from build123d import *

# Parameters (mm, degrees)
CROQUIS1_R              = 7.9
SALIENTE_EXTRUIR1_DEPTH = 7
CROQUIS2_R              = 6
SALIENTE_EXTRUIR2_DEPTH = 7.5
CROQUIS3_R              = 7.9
SALIENTE_EXTRUIR3_DEPTH = 1.5
CROQUIS4_R              = 4
CORTAR_EXTRUIR1_DEPTH   = 20.514609912
CROQUIS5_W              = 1.25
CROQUIS5_H              = 7.901
MATRIZC1_COUNT          = 2
MATRIZC1_ANGLE          = 90


with BuildPart() as part:
    # Croquis1 → Saliente-Extruir1 (new body)
    with BuildSketch(Plane(origin=(0, 0, 0), x_dir=(1, 0, 0), z_dir=(0, 1, 0))):
        with Locations(Location((0, 0, 0), (0, 0, 270))):
            Circle(CROQUIS1_R)
    extrude(amount=SALIENTE_EXTRUIR1_DEPTH)

    # Croquis2 → Saliente-Extruir2 (add)
    with BuildSketch(Plane(origin=(0, 7, 0), x_dir=(1, 0, 0), z_dir=(0, 1, 0))):
        with Locations(Location((0, 0, 0), (0, 0, 270))):
            Circle(CROQUIS2_R)
    extrude(amount=SALIENTE_EXTRUIR2_DEPTH)

    # Croquis3 → Saliente-Extruir3 (add)
    with BuildSketch(Plane(origin=(0, 14.5, 0), x_dir=(1, 0, 0), z_dir=(0, 1, 0))):
        with Locations(Location((0, 0, 0), (0, 0, 270))):
            Circle(CROQUIS3_R)
    extrude(amount=SALIENTE_EXTRUIR3_DEPTH)

    # Croquis4 → Cortar-Extruir1 (cut, through all)
    with BuildSketch(Plane(origin=(0, 16, 0), x_dir=(1, 0, 0), z_dir=(0, 1, 0))):
        with Locations(Location((0, 0, 0), (0, 0, 270))):
            Circle(CROQUIS4_R)
    extrude(amount=-CORTAR_EXTRUIR1_DEPTH, mode=Mode.SUBTRACT)

    # Croquis5 → Taladro roscado M31 (definir posicio) (revolve, cut)
    with BuildSketch(Plane(origin=(0, 3.5, 0), x_dir=(0, 1, 0), z_dir=(1, 0, 0))):
        with Locations((0.625, 3.9505)):
            Rectangle(CROQUIS5_W, CROQUIS5_H)
    taladro_roscado_m31_definir_posicio = revolve(axis=Axis((0, 3.5, -6.35), (0, 0, 1)), mode=Mode.SUBTRACT)

    # MatrizC1: Taladro roscado M31 (definir posicio) ×2 about axis
    matrizc1_axis = Axis((0, 7, 0), (0, -1, 0))
    for i in range(1, MATRIZC1_COUNT):
        add(taladro_roscado_m31_definir_posicio.rotate(matrizc1_axis, i * MATRIZC1_ANGLE / (MATRIZC1_COUNT - 1)), mode=Mode.SUBTRACT)


solid = part.part
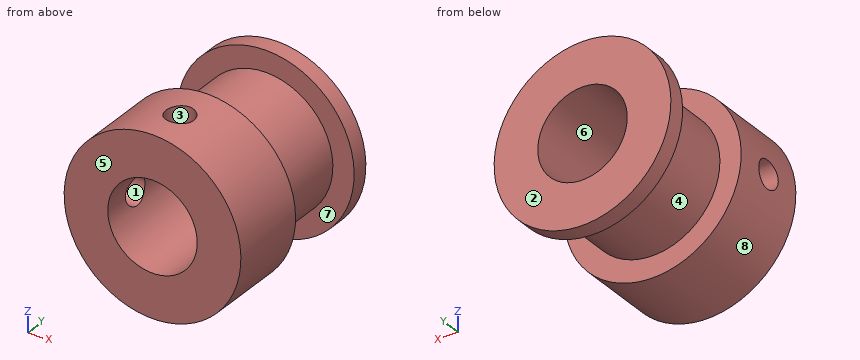
Here's how the part is built. I have some questions about the finished solid (model axes, mm). Face numbers are marked on the shaded views. A direction names the side the tool comes from. Round coordinates to 2 decimals unless told otherwise and drop trailing zeros. Loops run counter-clockwise (first coordinate to the right, second up) from the corner with the lowest first, then second, coordinate; pieces in that order, holes last. Notation, with made-up numbers: M -20.75,34.25 L -15.75,34.25 A23 ccw -15.75,57.25 Z; hole C 22,6 d4. An arc over 180 degrees is marked long. Write each question's results on one line, items separated by ' | '. Start each with the question number.
(1) Thinking about a two-plate mould opening in Z: for the marked faces 6, 7 and 8, which applies, pulls with the +Z half, pulls with the -Z half, needs draft (parallel to the pull), parting line crosses it, or undercut?
(2) I want a section at C-C (z = 0). Please give me the cut outline in (x, y).
(3) On a 3-axis mill with a long thin cutter (end or side, diameter ignored), from which of +Z, -Z, +X, -X, +Y, -Y can I reach the whole of each face in a straight line? I mean the marked faces 1, 2, 3, 4 and 5. Say none if no direction works.
(4) I want a section at B-B (z = 7.25). Please give me the cut outline in (x, y), then the cut area to 3 significant figures.
(5) I want a section at A-A (x = 0). Please give me the cut outline in (y, z), then the cut area to 4 significant figures.
(6) I want a section at D-D (y = 3.5). Please give me the cut outline in (x, z), then the cut area to 3 significant figures.
(7) Will these pins go through, and if not, where does the flat tip stop? P1, Ø8, axis at y = 11.5, z = -3, coming from the -X side; P2, Ø8, axis at x = -2, z = 0, coming from the +Y side; P3, Ø1.5, axis at x = 5, y = 9, coming from the -Z side; P4, Ø1.5, axis at x = 1, y = 5, coming from the +Z side.
(8) If I drill on probe 1 along X at (y, z) = (10.25, 0); probe 2 along Y at (x, z) = (7, 1.5); probe 3 along X at (y, z) = (3.5, 6.25), over which ranges is the centre line in solid material (lowest first)? Write a range as from..to.
Solved:
1) face 6: undercut | face 7: needs draft | face 8: parting line crosses it
2) outline: M -7.9,0 L -4,0 L -4,2.25 L -7.9,2.25 Z; M -7.9,4.75 L -4,4.75 L -4,16 L -7.9,16 L -7.9,14.5 L -6,14.5 L -6,7 L -7.9,7 Z; M 4,0 L 7.9,0 L 7.9,7 L 6,7 L 6,14.5 L 7.9,14.5 L 7.9,16 L 4,16 Z
3) face 1: -X | face 2: +Z, -Z, +X, -X, +Y | face 3: +Z | face 4: none | face 5: +Z, -Z, +X, -X, -Y
4) outline: M -3.14,0 L 3.14,0 L 3.14,7 L -3.14,7 Z; M -3.14,14.5 L 3.14,14.5 L 3.14,16 L -3.14,16 Z; hole C 0,3.5 d2.5 | area: 48.4 mm²
5) outline: M 0,-7.9 L 7,-7.9 L 7,-6 L 14.5,-6 L 14.5,-7.9 L 16,-7.9 L 16,-4 L 0,-4 Z; M 0,4 L 2.25,4 L 2.25,7.9 L 0,7.9 Z; M 4.75,4 L 16,4 L 16,7.9 L 14.5,7.9 L 14.5,6 L 7,6 L 7,7.9 L 4.75,7.9 Z | area: 86.55 mm²
6) outline: M -7.8,-1.25 A7.9 ccw long 1.25,7.8 L 1.25,3.8 A4 cw long -3.8,-1.25 Z; M -7.8,1.25 L -3.8,1.25 A4 cw -1.25,3.8 L -1.25,7.8 A7.9 ccw Z | area: 126 mm²
7) P1: stops at x = -7.89 | P2: stops at y = 16 | P3: stops at z = -4.24 | P4: stops at z = 7.9
8) probe 1: x = -6..-4, 4..6 | probe 2: y = 0..7, 14.5..16 | probe 3: x = -4.83..-1.25, 1.25..4.83
